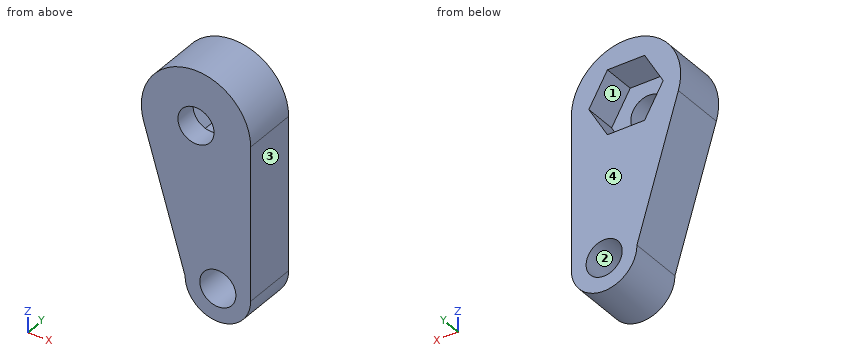
```python
from build123d import *

# Parameters (mm, degrees)
SKETCH1_R           = 1.65
BOSS_EXTRUDE1_DEPTH = 5
CUT_EXTRUDE1_DEPTH  = 3


with BuildPart() as part:
    # Sketch1 → Boss-Extrude1 (new body)
    with BuildSketch(Plane(origin=(0, 0, 0), x_dir=(1, 0, 0), z_dir=(0, 1, 0))):
        with BuildLine():
            Line((-1.123874335, 7.64724342), (-4.910860932, -4.908083254))
            ThreePointArc((-4.910860932, -4.908083254), (-0.85362327, -11.298412816), (4.876125665, -6.35195282))
            Line((4.876125665, -6.35195282), (4.876125665, 7.64724342))
            ThreePointArc((4.876125665, 7.64724342), (1.876125665, 10.64724342), (-1.123874335, 7.64724342))
        make_face()
        with Locations(Location((1.876125665, 7.64724342, 0), (0, 0, 270))):
            Circle(SKETCH1_R, mode=Mode.SUBTRACT)
        with Locations(Location((-0.123874335, -6.35195282, 0), (0, 0, 270))):
            Circle(SKETCH1_R, mode=Mode.SUBTRACT)
    extrude(amount=BOSS_EXTRUDE1_DEPTH)

    # Sketch2 → Cut-Extrude1 (cut)
    with BuildSketch(Plane(origin=(0, 5, 0), x_dir=(1, 0, 0), z_dir=(0, 1, 0))):
        Polygon((3.276125665, -6.352756866), (1.576821989, -3.40786847), (-1.823178011, -3.407064424), (-3.523874335, -6.351148774), (-1.82457066, -9.29603717), (1.57542934, -9.296841216), align=None)
    extrude(amount=-CUT_EXTRUDE1_DEPTH, mode=Mode.SUBTRACT)


solid = part.part
```
Part model, mm, in its own coordinate system. Face numbers are marked on the shaded views. Round coordinates to 2 decimals unless told otherwise and drop trailing zeros. Order: outer loops, then holes, each group sorted by start corner. A loop starts at its lowest first (then second) coordinate and runs counter-clockwise, first axis right, second up. Notation, with made-up numbers: M 3.25,66.25 L 14.25,66.25 A23 cw 14.25,98.25 Z; hole C -34,70.5 d5. An arc over 180 degrees is marked long. Answer in a Markdown table with one row per item. Add a question column.
Q1. Cut at B-B on z = -9. Give the cut face in (x, y).
Q2. Mould opens along X. For the marked faces 1, 2, 3 and 4 say: +X half, -X half, draft (parallel to the pull), parting line (faces both ways), or undercut.
Q3. Cut at C-C on y = 1.6. Give the cut face in (x, z), and give its area (3 significant figures).
Q4. Pin check, flat tips, straight feed: pin 1 (0.9 mm diameter, centred on x = 0.5, y = 3.5, fed in from +Z); pin 2 (1.8 mm diameter, centred on x = 1, z = 7.5, fed in from +Y); pin 3 (2.5 mm diameter, centred on x = 0, y = 3.5, fed in from -Z). Stop position of each tip, or through.
Q5. Wall check: L1, parallel to Z at x = 2.5, y = 4.05; L2, parallel to Z at x = 1.25, y = 1.35; L3, parallel to Z at x = 3, y = 0.4. Give the ranges that are in metal, low to high. Write a range as from..to.
Q6. Cut at A-A on x = 0.5. Give the cut face in (y, z).
Q7. Cut at D-D on x = -2.5. Give the cut face in (y, z).
Established:
| question | item | result |
|---|---|---|
| 1 | outline | M -0.8,0 L 0.93,0 L 0.93,5 L -0.8,5 Z; M 2.82,0 L 4.55,0 L 4.55,5 L 2.82,5 Z |
| 2 | face 1 | undercut |
| 2 | face 2 | undercut |
| 2 | face 3 | +X half |
| 2 | face 4 | draft |
| 3 | outline | M -4.91,4.91 L -1.12,-7.65 A3 ccw 4.88,-7.65 L 4.88,6.35 A5 ccw long Z; hole C -0.12,6.35 d3.3; hole C 1.88,-7.65 d3.3 |
| 3 | area | 150 mm2 |
| 4 | pin 1 | stops at z = 11.35 |
| 4 | pin 2 | stops at y = 2 |
| 4 | pin 3 | stops at z = -10.58 |
| 5 | L1 | z = -10.58..-9.17, -6.12..5.01, 7.7..10.61 |
| 5 | L2 | z = -10.58..-9.17, -6.12..5.44, 7.27..11.16 |
| 5 | L3 | z = -10.43..-8.86, -6.44..10.26 |
| 6 | outline | M 0,-10.31 L 5,-10.31 L 5,-8.56 L 0,-8.56 Z; M 0,-6.74 L 5,-6.74 L 5,3.41 L 2,3.41 L 2,4.82 L 0,4.82 Z; M 0,7.88 L 2,7.88 L 2,9.3 L 5,9.3 L 5,11.31 L 0,11.31 Z |
| 7 | outline | M 0,-3.08 L 5,-3.08 L 5,4.58 L 2,4.58 L 2,8.13 L 5,8.13 L 5,10.75 L 0,10.75 Z |
